```python
from build123d import *

# Parameters (mm, degrees)
F1_DEPTH  = 38.1
F3_R      = 30.2729737571
F4_DEPTH  = 94.742
F5_W      = 180.7619705796
F5_H      = 196.721881628
F6_DEPTH  = 25.4
F7_DEPTH  = 107.1100030094
F8_R      = 5
F9_SIZE   = 5
F11_W     = 170.7619705796
F11_H     = 186.721881628
F11_R     = 11.555445332
F11_R_2   = 13.3506180186
F12_DEPTH = 25


with BuildPart() as f1:
    # F0 (on Front) → F1 (new body)
    with BuildSketch(Plane.XZ):
        Polygon((34.2515595257, -19.7751471123), (34.2515595257, 19.7751471123), (0, 39.5502942247), (-34.2515595257, 19.7751471123), (-34.2515595257, -19.7751471123), (0, -39.5502942247), align=None)
    extrude(amount=F1_DEPTH)

    # F3 (on face) → F4 (cut)
    with BuildSketch(Plane(origin=(0, 0, 0), x_dir=(-1, 0, 0), z_dir=(0, 1, 0))):
        Circle(F3_R)
    extrude(amount=-F4_DEPTH, mode=Mode.SUBTRACT)

    # F5 (on Front) → F6 (join)
    with BuildSketch(Plane.XZ):
        with Locations((0.411581248, 3.1727701426)):
            Rectangle(F5_W, F5_H)
    extrude(amount=F6_DEPTH)

    # F7 (cut): a face of the model
    f7_faces = [f1.faces().sort_by_distance(p)[0] for p in [
        (0, -25.4, 0),
    ]]
    extrude(f7_faces, amount=-F7_DEPTH, mode=Mode.SUBTRACT)

    # F8
    f8_edges = [f1.edges().sort_by_distance(p)[0] for p in [
        (17.12578, -25.4, 29.662721),
        (-17.12578, -25.4, 29.662721),
        (34.25156, -25.4, 0),
        (17.12578, -25.4, -29.662721),
        (-17.12578, -25.4, -29.662721),
        (-34.25156, -25.4, 0),
    ]]
    fillet(f8_edges, radius=F8_R)

    # F9
    f9_edges = [f1.edges().sort_by_distance(p)[0] for p in [
        (90.792567, -12.7, 101.533711),
        (19.62578, -25.4, 33.992848),
        (39.25156, -25.4, 0),
        (-19.62578, -25.4, 33.992848),
        (19.62578, -25.4, -33.992848),
        (-39.25156, -25.4, 0),
        (-19.62578, -25.4, -33.992848),
        (0.411581, -25.4, 101.533711),
        (90.792567, -25.4, 3.17277),
        (-89.969404, -25.4, 3.17277),
        (0.411581, -25.4, -95.188171),
        (-89.969404, -12.7, 101.533711),
        (-89.969404, -12.7, -95.188171),
        (90.792567, -12.7, -95.188171),
    ]]
    chamfer(f9_edges, length=F9_SIZE)

    # F11 (on face) → F12 (join)
    with BuildSketch(Plane.XZ.offset(25.4)):
        with Locations((0.411581248, 3.1727701426)):
            Rectangle(F11_W, F11_H)
        Polygon((-39.2515595257, -22.6618984583), (-39.2515595257, 22.6618984583), (0, 45.3237969166), (39.2515595257, 22.6618984583), (39.2515595257, -22.6618984583), (0, -45.3237969166), align=None, mode=Mode.SUBTRACT)
        with Locations((-56.5757006407, 60.9375908971)):
            Circle(F11_R, mode=Mode.SUBTRACT)
        with Locations((51.4449626207, 60.9523579478)):
            Circle(F11_R_2, mode=Mode.SUBTRACT)
    extrude(amount=F12_DEPTH)


solid = f1.part
```
Design review of the part built by this model. Coordinates are the model's own, in mm. A direction names the side the tool comes from. Give positions to 0.01 mm unless a question says otherwise; leave off trailing zeros. Write each loop counter-clockwise with the first axis right and the second up, starting at its lowest first coordinate (ties: lowest second). Pieces come first, ordered by that corner, then holes. Notation, with made-up numbers: (53, 89.5) -> (72, 89.5) arc R21 ccw to (72, 118.5) -> close; hole circle Ø5 at (-11, -30). An arc over 180 degrees is marked (long way). Answer in a Markdown table with one row per item.
(1) For faces 1 (the flat face through (-1, -38, 96.534)), 2 (the cylindrical face through (41.61, -37.72, 69.98)), 3 (the flat face through (-84.969, -38, 2)), list the 3-axis set-ups (+Z, -Z, +X, -X, +Y, -Y) from which the entire face can be reached by the end or side of a thin tool; tool diameter is ignored.
Results:
| item | result |
|---|---|
| face 1 | +Z, +X, -X, -Y |
| face 2 | -Y |
| face 3 | +Z, -Z, -X, -Y |
(2) Consider section C-C (z = -61). State the section outline as (x, y) points, then the cut area to 3 significant figures.
Results:
| item | result |
|---|---|
| outline | (-89.97, -20.4) -> (-84.97, -25.4) -> (-84.97, -50.4) -> (85.79, -50.4) -> (85.79, -25.4) -> (90.79, -20.4) -> (90.79, 0) -> (-89.97, 0) -> close |
| area | 8,840 mm2 |
(3) Mouldability with a two-part tool opening along Z and no side actions: class faces 4 (the flat face through (88.33, -10.06, -92.65)), 5 (the flat face through (34.252, -34, 0)), 6 (the flat face through (88.328, -22.865, 1.866)) as +Z half, -Z half, draft (parallel to the pull), parting line (faces both ways), or undercut.
Results:
| item | result |
|---|---|
| face 4 | -Z half |
| face 5 | undercut |
| face 6 | draft |
(4) Clearance check with flat-ended pins moving along their axes: pin 1 (7.5 mm diameter, centred on y = -41.5, z = -2.5, fed in from +X); pin 2 (12 mm diameter, centred on x = 64.5, y = -29, fed in from -Z); pin 3 (7 mm diameter, centred on x = -57, z = 62, fed in from -Y); pin 4 (4 mm diameter, centred on x = 66, z = 48.5, fed in from +Y). State where each tip first meets the part, or that it passes through.
Results:
| item | result |
|---|---|
| pin 1 | x = 85.79 |
| pin 2 | z = -92.59 |
| pin 3 | y = -25.4 |
| pin 4 | y = 0 |
(5) To check wall thickness, follow probe 1 along Z at (x, y) = (0, -31); probe 2 along X at (y, z) = (-47.5, -13); probe 3 along Z at (x, y) = (1, -37). State the ranges of each line that lie inside material, in increasing order.
Results:
| item | result |
|---|---|
| probe 1 | -90.19 to -45.32, -39.55 to -30.27, 30.27 to 39.55, 45.32 to 96.53 |
| probe 2 | -84.97 to -39.25, 39.25 to 85.79 |
| probe 3 | -90.19 to -44.75, -38.97 to -30.26, 30.26 to 38.97, 44.75 to 96.53 |
(6) Consider section A-A (z = 0). State the section outline as (x, y) points.
Results:
| item | result |
|---|---|
| outline | (-89.97, -20.4) -> (-84.97, -25.4) -> (-84.97, -50.4) -> (-39.25, -50.4) -> (-39.25, -25.4) arc R5 cw to (-34.25, -30.4) -> (-34.25, -38.1) -> (-30.27, -38.1) -> (-30.27, 0) -> (-89.97, 0) -> close; (30.27, -38.1) -> (34.25, -38.1) -> (34.25, -30.4) arc R5 cw to (39.25, -25.4) -> (39.25, -50.4) -> (85.79, -50.4) -> (85.79, -25.4) -> (90.79, -20.4) -> (90.79, 0) -> (30.27, 0) -> close |
(7) Consider section D-D (y = -15). State the section outline as (x, z) points, then the cut area to 3 significant figures.
Results:
| item | result |
|---|---|
| outline | (-89.97, -90.19) -> (-84.97, -95.19) -> (85.79, -95.19) -> (90.79, -90.19) -> (90.79, 96.53) -> (85.79, 101.53) -> (-84.97, 101.53) -> (-89.97, 96.53) -> close; hole circle Ø60.55 at (0, 0) |
| area | 32,600 mm2 |
(8) Consider section B-B (x = 77.5). State the section outline as (y, z) points, then the cut area to 3 significant figures.
Results:
| item | result |
|---|---|
| outline | (-50.4, -90.19) -> (-25.4, -90.19) -> (-20.4, -95.19) -> (0, -95.19) -> (0, 101.53) -> (-20.4, 101.53) -> (-25.4, 96.53) -> (-50.4, 96.53) -> close |
| area | 9,640 mm2 |
